from build123d import *

# Parameters (mm, degrees)
SZKIC1_W                    = 36
SZKIC1_H                    = 16
DODANIE_WYCI_GNI_CIE1_DEPTH = 10
WYTNIJ_WYCI_GNI_CIE1_DEPTH  = 10
SZKIC3_R                    = 1.55
WYTNIJ_WYCI_GNI_CIE2_DEPTH  = 74.950499929
SZKIC4_W                    = 6.55
SZKIC4_H                    = 10
DODANIE_WYCI_GNI_CIE2_DEPTH = 6
SZKIC5_W                    = 6.55
SZKIC5_H                    = 10
DODANIE_WYCI_GNI_CIE3_DEPTH = 10


with BuildPart() as part:
    # Szkic1 → Dodanie-wyciągnięcie1 (new body)
    with BuildSketch(Plane.XY):
        with Locations((53.502982034, -8)):
            Rectangle(SZKIC1_W, SZKIC1_H)
    extrude(amount=-DODANIE_WYCI_GNI_CIE1_DEPTH)

    # Szkic2 → Wytnij-wyciągnięcie1 (cut)
    with BuildSketch(Plane(origin=(0, 0, -10), x_dir=(-1, 0, 0), z_dir=(0, 0, -1))):
        with BuildLine():
            Line((-57.391426453, -16), (-49.614537615, -16))
            Line((-49.614537615, -16), (-49.614537615, -14.730541148))
            Line((-49.614537615, -14.730541148), (-49.204397396, -15.128067711))
            ThreePointArc((-49.204397396, -15.128067711), (-53.507441674, -4.70000163), (-57.795233679, -15.134348373))
            Line((-57.795233679, -15.134348373), (-57.391426453, -14.730541148))
            Line((-57.391426453, -14.730541148), (-57.391426453, -16))
        make_face()
    extrude(amount=-WYTNIJ_WYCI_GNI_CIE1_DEPTH, mode=Mode.SUBTRACT)

    # Szkic3 → Wytnij-wyciągnięcie2 (cut, through all)
    with BuildSketch(Plane(origin=(0, 0, -10), x_dir=(-1, 0, 0), z_dir=(0, 0, -1))):
        with Locations((-44.502982034, -12)):
            Circle(SZKIC3_R)
        with Locations((-44.502982034, -4)):
            Circle(SZKIC3_R)
        with Locations((-62.502982034, -12)):
            Circle(SZKIC3_R)
        with Locations((-62.502982034, -4)):
            Circle(SZKIC3_R)
    extrude(amount=-WYTNIJ_WYCI_GNI_CIE2_DEPTH, mode=Mode.SUBTRACT)

    # Szkic4 → Dodanie-wyciągnięcie2 (add)
    with BuildSketch(Plane.XZ.offset(16)):
        with Locations((68.227982034, -5)):
            Rectangle(SZKIC4_W, SZKIC4_H)
        with Locations((38.777982035, -5)):
            Rectangle(SZKIC4_W, SZKIC4_H)
    extrude(amount=DODANIE_WYCI_GNI_CIE2_DEPTH)

    # Szkic5 → Dodanie-wyciągnięcie3 (add)
    with BuildSketch(Plane(origin=(0, 0, 0), x_dir=(1, 0, 0), z_dir=(0, 1, 0))):
        with Locations((68.227982034, 5)):
            Rectangle(SZKIC5_W, SZKIC5_H)
        with Locations((38.777982035, 5)):
            Rectangle(SZKIC5_W, SZKIC5_H)
    extrude(amount=DODANIE_WYCI_GNI_CIE3_DEPTH)


solid = part.part
Here's how the part is built. I have some questions about the finished solid (model axes, mm). A direction names the side the tool comes from. Round coordinates to 2 decimals unless told otherwise and drop trailing zeros. Order: outer loops, then holes, each group sorted by start corner. A loop starts at its lowest first (then second) coordinate and runs counter-clockwise, first axis right, second up. Notation, with made-up numbers: M 38.5,67 L 67.5,67 A26 cw 67.5,105 Z; hole C 34,85 d6. An arc over 180 degrees is marked long. Return JSON: item names as keys, results as strings. Group by question number.
1. On a 3-axis mill with a long thin cutter (end or side, diameter ignored), from which of +Z, -Z, +X, -X, +Y, -Y can I reach the whole of each face in a straight line? I mean faces 4 (the face through (42.053, 5, -5)), 5 (the face through (57.391, -15, -5)), 6 (the face through (43.025, -3.534, -5.07)). Say none if no direction works.
2. If we mould it in two halves opening along X, with no side actions, what happens to faces 1 (the face through (35.503, -6, -5)), 2 (the face through (53, -3, -10)), 3 (the face through (64.953, -19, -5))? For each: pulls with the +X half, pulls with the -X half, needs draft (parallel to the pull), parting line crosses it, or undercut.
3. I'm going to push flat-ended pins straight in: pin 1 Ø4 at (x, z) = (61.5, -2) entering from +Y; pin 2 Ø2.5 at (x, y) = (62.5, -12) entering from -Z; pin 3 Ø5 at (x, y) = (44.5, -12) entering from -Z; pin 4 Ø2.5 at (x, z) = (62, -2.5) entering from -Y. Where does each tip first touch, or does it pass through?
4. If we section it at D-D on z = -3.75: List the corners of the cut face in (x, y) for me.
5. Please list where these lines run through material, in increasing order: probe 1 along Y at (x, z) = (62.5, -8.5); probe 2 along X at (y, z) = (-18, -9); probe 3 along X at (y, z) = (-10.8, -2.5).
6. If we section it at B-B on x = 62.5: List the corners of the cut face in (y, z) for me, then the cut area to 3 significant figures.
7. If we section it at C-C on y = -4: List the corners of the cut face in (x, z) for me, then the cut area to 3 significant figures.
8. If we section it at A-A on y = 6.5: List the corners of the cut face in (x, z) for me, then the cut area to 3 significant figures.
Reply:
{
 "1": {"face 4": "+Z, -Z, +Y", "face 5": "+Z, -Z, -Y", "face 6": "+Z, -Z"},
 "2": {"face 1": "pulls with the -X half", "face 2": "needs draft", "face 3": "undercut"},
 "3": {"pin 1": "y = 0", "pin 2": "through", "pin 3": "z = -10", "pin 4": "y = -16"},
 "4": {"outline": "M 35.5,-22 L 42.05,-22 L 42.05,-16 L 49.61,-16 L 49.61,-14.73 L 49.2,-15.13 A6.1 cw long 57.8,-15.13 L 57.39,-14.73 L 57.39,-16 L 64.95,-16 L 64.95,-22 L 71.5,-22 L 71.5,10 L 64.95,10 L 64.95,0 L 42.05,0 L 42.05,10 L 35.5,10 Z; hole C 44.5,-12 d3.1; hole C 44.5,-4 d3.1; hole C 62.5,-12 d3.1; hole C 62.5,-4 d3.1"},
 "5": {"probe 1": "-16 to -13.55, -10.45 to -5.55, -2.45 to 0", "probe 2": "35.5 to 42.05, 64.95 to 71.5", "probe 3": "35.5 to 43.52, 45.48 to 47.4, 59.6 to 61.52, 63.48 to 71.5"},
 "6": {"outline": "M -16,-10 L -13.55,-10 L -13.55,0 L -16,0 Z; M -10.45,-10 L -5.55,-10 L -5.55,0 L -10.45,0 Z; M -2.45,-10 L 0,-10 L 0,0 L -2.45,0 Z", "area": "98.0 mm^2"},
 "7": {"outline": "M 35.5,-10 L 42.95,-10 L 42.95,0 L 35.5,0 Z; M 46.05,-10 L 60.95,-10 L 60.95,0 L 46.05,0 Z; M 64.05,-10 L 71.5,-10 L 71.5,0 L 64.05,0 Z", "area": "298 mm^2"},
 "8": {"outline": "M 35.5,-10 L 42.05,-10 L 42.05,0 L 35.5,0 Z; M 64.95,-10 L 71.5,-10 L 71.5,0 L 64.95,0 Z", "area": "131 mm^2"}
}
